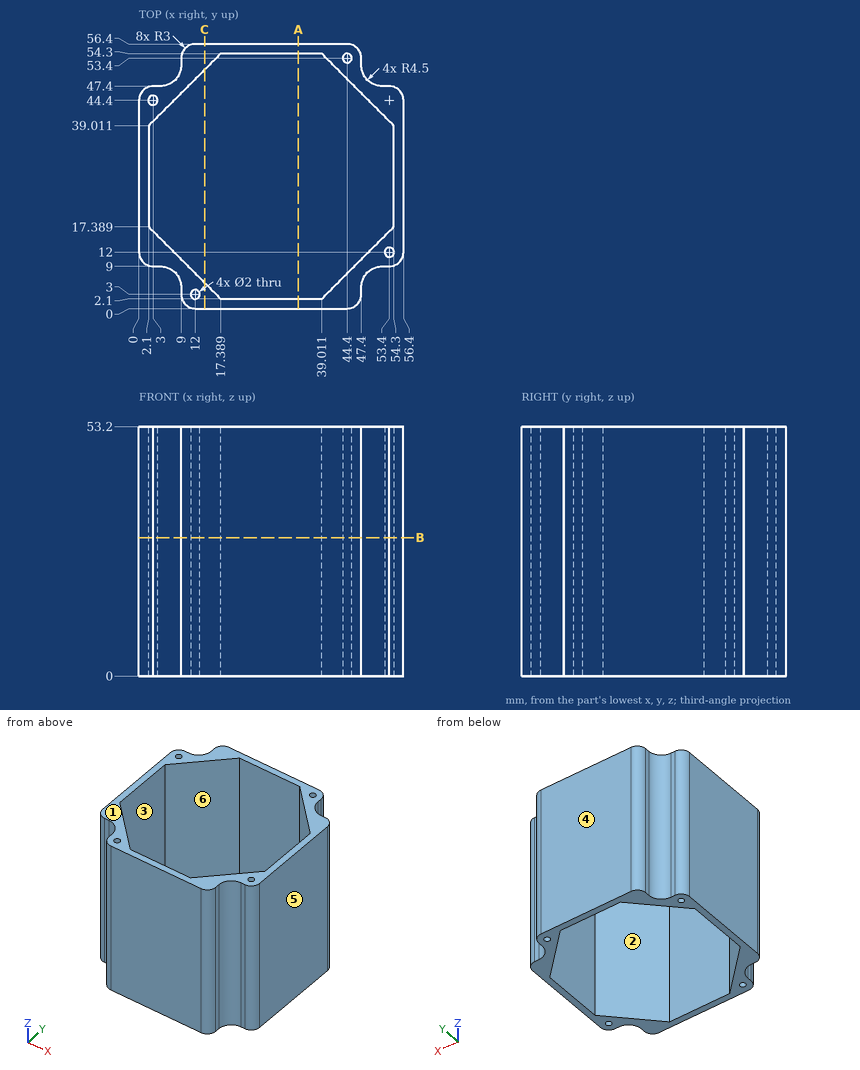
Geometry check sheet. Reference: drawing and pictorial views, mm from the part's lowest x, y, z. A direction names the side the tool comes from. Coordinates: 2 decimals unless noted, no trailing zeros. Order: outer loops, then holes, each group sorted by start corner. A loop starts at its lowest first (then second) coordinate and runs counter-clockwise, first axis right, second up.
Item 1: Section check B-B, the plane z = 29.5. Give the number of separate pieces and of enclosed holes in the cut face, then the cut area to 3 significant figures.
Filled in:
separate pieces: 1
enclosed holes: 5
area: 589 mm2
Item 2: Depth check by flat-ended pin: pin 1 (6 mm diameter, centred on x = 50, z = 11.5, fed in from -Y); pin 2 (1.6 mm diameter, centred on x = 44.4, y = 53.4, fed in from -Z); pin 3 (1.2 mm diameter, centred on y = 3.5, z = 28.5, fed in from -X); pin 4 (1.2 mm diameter, centred on x = 53, z = 20.5, fed in from -Y). Enter the tip coordinate at first touch or a pass-through.
Filled in:
pin 1: stops at y = 1.5
pin 2: passes through
pin 3: stops at x = 9
pin 4: stops at y = 9
Item 3: Material ranges on L1, parallel to X at y = 32, z = 37; L2, parallel to Y at x = 53, z = 39, recorded low to high.
Filled in:
L1: x = 0 to 2.1, 54.3 to 56.4
L2: y = 9 to 11.08, 12.92 to 16.09, 40.31 to 47.4
Item 4: Section check A-A, the plane x = 34. Enter the section's corners in (y, z), then the cut area to 3 significant figures.
Filled in:
outline: (0, 0) - (2.1, 0) - (2.1, 53.2) - (0, 53.2) - close; (54.3, 0) - (56.4, 0) - (56.4, 53.2) - (54.3, 53.2) - close
area: 223 mm2
Item 5: Section check C-C, the plane x = 14. Enter the section's corners in (y, z).
Filled in:
outline: (0, 0) - (5.49, 0) - (5.49, 53.2) - (0, 53.2) - close; (50.91, 0) - (56.4, 0) - (56.4, 53.2) - (50.91, 53.2) - close
Item 6: Release check for a two-part mould opening along X. For the marked faces 3, 4, 5 and 6 record: +X half, -X half, draft (parallel to the pull), parting line (faces both ways), or undercut.
Filled in:
face 3: undercut
face 4: draft
face 5: +X half
face 6: undercut
Item 7: Access from +Z, -Z, +X, -X, +Y, -Y to the whole of each face (thin tool, end or side, straight path). Record for the marked faces 1 and 2.
Filled in:
face 1: +Z, +X, -X, +Y, -Y
face 2: +Z, -Z
